```python
from build123d import *

# Parameters (mm, degrees)
SKETCH2_R               = 2.75
SKETCH3_R               = 2.75
SKETCH3_7_W             = 10
SKETCH3_7_H             = 10
BOSS_EXTRUDE4_DEPTH     = 4
SKETCH8_W               = 1.7
SKETCH8_H               = 8.5
CUT_EXTRUDE2_DEPTH      = 1
CUT_EXTRUDE2_DEPTH_BACK = 11
FILLET1_R               = 1
SKETCH11_R              = 1.25
CUT_EXTRUDE4_DEPTH      = 6
CUT_EXTRUDE4_DEPTH_BACK = 6


with BuildPart() as part:
    # Sketch2 → Loft1 section 0
    with BuildSketch(Plane.XY):
        Circle(SKETCH2_R)
    # Sketch3 → Loft1 section 1
    with BuildSketch(Plane.XY.offset(25)):
        Circle(SKETCH3_R)
    loft()

    # Sketch3<7> → Boss-Extrude4 (add)
    with BuildSketch(Plane.XY.offset(25)):
        Rectangle(SKETCH3_7_W, SKETCH3_7_H)
    extrude(amount=BOSS_EXTRUDE4_DEPTH)

    # Sketch8 → Cut-Extrude2 (cut, two sides)
    with BuildSketch(Plane(origin=(5, 0, 0), x_dir=(0, 0, -1), z_dir=(1, 0, 0))) as cut_extrude2_sk:
        with Locations((-27, 0)):
            Rectangle(SKETCH8_W, SKETCH8_H)
    extrude(amount=CUT_EXTRUDE2_DEPTH, mode=Mode.SUBTRACT)
    extrude(cut_extrude2_sk.sketch, amount=-CUT_EXTRUDE2_DEPTH_BACK, mode=Mode.SUBTRACT)

    # Fillet1
    fillet1_edges = [part.edges().sort_by_distance(p)[0] for p in [
        (-2.75, 0, 25),
    ]]
    fillet(fillet1_edges, radius=FILLET1_R)

    # Sketch11 → Cut-Extrude4 (cut, two sides)
    with BuildSketch(Plane(origin=(0, 0, 0), x_dir=(0, 0, -1), z_dir=(1, 0, 0))) as cut_extrude4_sk:
        with Locations((-12, 0)):
            Circle(SKETCH11_R)
    extrude(amount=CUT_EXTRUDE4_DEPTH, mode=Mode.SUBTRACT)
    extrude(cut_extrude4_sk.sketch, amount=-CUT_EXTRUDE4_DEPTH_BACK, mode=Mode.SUBTRACT)


solid = part.part
```
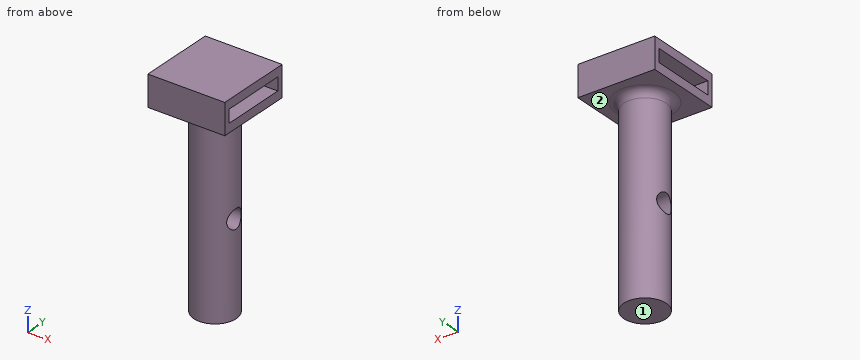
Geometry check sheet. Reference: the model listing, model coordinates, mm. Face numbers are marked on the shaded views. A direction names the side the tool comes from. Coordinates: 2 decimals unless noted, no trailing zeros. Write each loop counter-clockwise with the first axis right and the second up, starting at its lowest first coordinate (ties: lowest second). Pieces come first, ordered by that corner, then holes. Notation, with made-up numbers: (-0.75, 0) -> (49.25, 0) arc R15 cw to (49.25, 23) -> close; hole circle Ø5 at (37.25, 62). An arc over 180 degrees is marked (long way). Use CSV: the item, a comma, the result in double quotes. Start each with the question number.
Item 1: Cross-section at B-B, the plane x = 1. State how many separate pieces and enclosed holes the cut face has, plus the area to 3 significant figures.
Item 2: Thickness scan on line 1 (Z direction, x = 1.85, y = 0); line 2 (Z direction, x = -3.5, y = 4); line 3 (Z direction, x = -1.25, y = -1.75). Record the ranges inside material, lowest first.
Item 3: Depth check by flat-ended pin: pin 1 Ø2 at (x, z) = (-4, 3.5) entering from -Y; pin 2 Ø3 at (y, z) = (0, 12) entering from -X; pin 3 Ø3 at (y, z) = (0, 12) entering from +X; pin 4 Ø6 at (x, z) = (-4, 18) entering from +Y. Enter the tip coordinate at first touch or a pass-through.
Item 4: Cross-section at A-A, the plane z = 5. Record the cut outline in (x, y), plus the area to 3 significant figures.
Item 5: Cross-section at C-C, the plane z = 12. Record the cut outline in (x, y), plus the area to 3 significant figures.
Item 6: Set-up check for the marked faces 1 and 2: record each of +Z, -Z, +X, -X, +Y, -Y from which the full face is reachable in a straight line by a thin tool's end or side.
Answers:
1,separate pieces,"1"
1,enclosed holes,"2"
1,area,"149 mm^2"
2,line 1,"0 to 10.75, 13.25 to 26.15, 27.85 to 29"
2,line 2,"25 to 26.15, 27.85 to 29"
2,line 3,"0 to 26.15, 27.85 to 29"
3,pin 1,"through"
3,pin 2,"x = -2.75"
3,pin 3,"x = 2.75"
3,pin 4,"y = 2.56"
4,outline,"circle Ø5.5 at (0, 0)"
4,area,"23.8 mm^2"
5,outline,"(-2.45, -1.25) arc R2.75 ccw to (2.45, -1.25) -> close; (-2.45, 1.25) -> (2.45, 1.25) arc R2.75 ccw to start"
5,area,"10.5 mm^2"
6,face 1,"-Z, +X, -X, +Y, -Y"
6,face 2,"-Z"
